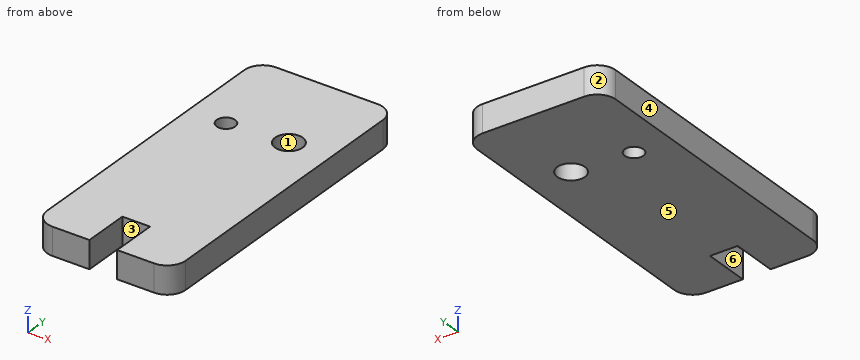
```python
from build123d import *

# Parameters (mm, degrees)
SKETCH1_R           = 1.5
SKETCH1_R_2         = 1
BOSS_EXTRUDE1_DEPTH = 3
SKETCH4_W           = 3
SKETCH4_H           = 5
CUT_EXTRUDE1_DEPTH  = 4


with BuildPart() as part:
    # Sketch1 → Boss-Extrude1 (new body)
    with BuildSketch(Plane.XY):
        with BuildLine():
            Line((2, 0), (13, 0))
            ThreePointArc((13, 0), (14.414213562, 0.585786438), (15, 2))
            Line((15, 2), (15, 32))
            ThreePointArc((15, 32), (14.414213562, 33.414213562), (13, 34))
            Line((13, 34), (2, 34))
            ThreePointArc((2, 34), (0.585786438, 33.414213562), (0, 32))
            Line((0, 32), (0, 2))
            ThreePointArc((0, 2), (0.585786438, 0.585786438), (2, 0))
        make_face()
        with Locations((10.521654895, 24)):
            Circle(SKETCH1_R, mode=Mode.SUBTRACT)
        with Locations((4.038452424, 23.533003519)):
            Circle(SKETCH1_R_2, mode=Mode.SUBTRACT)
    extrude(amount=BOSS_EXTRUDE1_DEPTH)

    # Sketch4 → Cut-Extrude1 (cut, through all)
    with BuildSketch(Plane.XY.offset(3)):
        with Locations((7.5, 2.5)):
            Rectangle(SKETCH4_W, SKETCH4_H)
    extrude(amount=-CUT_EXTRUDE1_DEPTH, mode=Mode.SUBTRACT)


solid = part.part
```
Here's how the part is built. I have some questions about the finished solid (model axes, mm). Face numbers are marked on the shaded views. A direction names the side the tool comes from. Coordinates: 2 decimals unless noted, no trailing zeros. Order: outer loops, then holes, each group sorted by start corner. A loop starts at its lowest first (then second) coordinate and runs counter-clockwise, first axis right, second up. Notation, with made-up numbers: (70, 2.25) - (92, 2.25) arc R20 cw to (92, 21.25) - close; hole circle Ø9 at (61, 33). An arc over 180 degrees is marked (long way). One line per question, with ' | ' between items.
(1) Will this pin go through, and if not, where does the flat tip stop? pin 1 (2 mm diameter, centred on x = 6.5, y = 14.5, fed in from -Z).
Report:
pin 1: stops at z = 0
(2) If we mould it in two halves opening along Y, with no side actions, what happens to the marked faces 1, 2, 3 and 4? For each: pulls with the +Y half, pulls with the -Y half, needs draft (parallel to the pull), parting line crosses it, or undercut.
Report:
face 1: undercut | face 2: pulls with the +Y half | face 3: pulls with the -Y half | face 4: needs draft
(3) Suppose I cut it at A-A on z = 2.1. List the corners of the cut face in (x, y) for me.
Report:
outline: (0, 2) arc R2 ccw to (2, 0) - (6, 0) - (6, 5) - (9, 5) - (9, 0) - (13, 0) arc R2 ccw to (15, 2) - (15, 32) arc R2 ccw to (13, 34) - (2, 34) arc R2 ccw to (0, 32) - close; hole circle Ø2 at (4.04, 23.53); hole circle Ø3 at (10.52, 24)
(4) If I drill on L1, parallel to Y at x = 7.5, z = 2.2; L2, parallel to Y at x = 11.75, z = 2; L3, parallel to Y at x = 3.75, z = 1.2, over which ranges is the centre line in solid material (lowest first)?
Report:
L1: y = 5 to 34 | L2: y = 0 to 23.14, 24.86 to 34 | L3: y = 0 to 22.58, 24.49 to 34
(5) Suppose I cut it at B-B on y = 24. List the corners of the cut face in (x, z) for me, and give its area (3 significant figures).
Report:
outline: (0, 0) - (3.15, 0) - (3.15, 3) - (0, 3) - close; (4.92, 0) - (9.02, 0) - (9.02, 3) - (4.92, 3) - close; (12.02, 0) - (15, 0) - (15, 3) - (12.02, 3) - close | area: 30.7 mm2
(6) For the marked faces 5 and 6, which set-ups out of +Z, -Z, +X, -X, +Y, -Y let a thin tool reach every point of the face, with its end or its side?
Report:
face 5: -Z, +X, -X, +Y, -Y | face 6: +Z, -Z, -Y
